```python
from build123d import *
from OCP.BRepAlgoAPI import BRepAlgoAPI_Cut
from OCP.TopTools import TopTools_ListOfShape

# Parameters (mm, degrees)
BOSS_EXTRUDE1_DEPTH = 75
FILLET1_R           = 2
SKETCH4_W           = 25.830037715
SKETCH4_H           = 76.964783177
CUT_EXTRUDE3_DEPTH  = 10
SKETCH7_W           = 75
SKETCH7_H           = 2.5
BOSS_EXTRUDE2_DEPTH = 7.180004
SKETCH9_W           = 2.5
SKETCH9_H           = 75
BOSS_EXTRUDE3_DEPTH = 20
SKETCH10_W          = 68.5
SKETCH10_H          = 2.5
BOSS_EXTRUDE4_DEPTH = 20
BOSS_EXTRUDE5_START = -67.82
BOSS_EXTRUDE5_DEPTH = 67.82
CUT_EXTRUDE4_DEPTH  = 7.32
SKETCH13_W          = 1.35
SKETCH13_H          = 15.1
CUT_EXTRUDE5_DEPTH  = 7.32
SKETCH15_R          = 1.15
CUT_EXTRUDE6_DEPTH  = 7.32
SKETCH16_R          = 1.15
CUT_EXTRUDE7_DEPTH  = 7.32
BOSS_EXTRUDE8_DEPTH = 59.999996
CHAMFER1_SIZE       = 0.75
CHAMFER2_SIZE       = 0.75


with BuildPart() as part:
    # Sketch1 → Boss-Extrude1 (new body)
    with BuildSketch(Plane(origin=(0, 0, 0), x_dir=(1, 0, 0), z_dir=(0, 1, 0))):
        with BuildLine():
            Line((-20.27294978, -55.394285714), (-17.826119678, -54.881428571))
            ThreePointArc((-17.826119678, -54.881428571), (-18.344064324, -51.565724334), (-18.517328344, -48.214285714))
            Line((-18.517328344, -48.214285714), (-18.517328344, 11.925714286))
            Line((-18.517328344, 11.925714286), (-5.357328344, 11.925714286))
            Line((-5.357328344, 11.925714286), (-5.357328344, 14.425714286))
            Line((-5.357328344, 14.425714286), (-21.017328344, 14.425714286))
            Line((-21.017328344, 14.425714286), (-21.017328344, -48.214285714))
            ThreePointArc((-21.017328344, -48.214285714), (-20.830736323, -51.823527305), (-20.27294978, -55.394285714))
        make_face()
    extrude(amount=BOSS_EXTRUDE1_DEPTH)

    # Fillet1
    fillet1_edges = [part.edges().sort_by_distance(p)[0] for p in [
        (-21.017328344, 37.5, -14.425714286),
        (-18.517328344, 37.5, -11.925714286),
    ]]
    fillet(fillet1_edges, radius=FILLET1_R)

    # Sketch4 → Cut-Extrude3 (cut)
    with BuildSketch(Plane(origin=(-18.517328344, 0, 0), x_dir=(0, 0, -1), z_dir=(1, 0, 0))):
        with Locations((-51.201481413, 38.482391589)):
            Rectangle(SKETCH4_W, SKETCH4_H)
    extrude(amount=CUT_EXTRUDE3_DEPTH, mode=Mode.SUBTRACT)

    # Sketch7 → Boss-Extrude2 (add)
    with BuildSketch(Plane(origin=(0, 0, 48.214285714), x_dir=(0, -1, 0), z_dir=(0, 0, 1))):
        with Locations((-37.5, -19.767328344)):
            Rectangle(SKETCH7_W, SKETCH7_H)
    extrude(amount=BOSS_EXTRUDE2_DEPTH)

    # Sketch9 → Boss-Extrude3 (add)
    with BuildSketch(Plane(origin=(-5.357328344, 0, 0), x_dir=(0, 0, -1), z_dir=(1, 0, 0))):
        with Locations((13.175714286, 37.5)):
            Rectangle(SKETCH9_W, SKETCH9_H)
    extrude(amount=BOSS_EXTRUDE3_DEPTH)

    # Sketch10 → Boss-Extrude4 (add)
    with BuildSketch(Plane(origin=(-18.517328344, 0, 0), x_dir=(0, 0, -1), z_dir=(1, 0, 0))):
        with Locations((-21.144285714, 73.75)):
            Rectangle(SKETCH10_W, SKETCH10_H)
    extrude(amount=BOSS_EXTRUDE4_DEPTH)

    # Sketch11 → Boss-Extrude5 (add)
    with BuildSketch(Plane.XY.offset(55.394285714).offset(BOSS_EXTRUDE5_START)):
        Polygon((-20.767328344, 0), (-18.767328344, 0), (-19.767328344, -2), align=None)
    extrude(amount=BOSS_EXTRUDE5_DEPTH)

    # Sketch12 → Cut-Extrude4 (cut)
    with BuildSketch(Plane.XY.offset(55.394285714)):
        Polygon((-20.767328344, 0), (-18.767328344, 0), (-19.767328344, -2), align=None)
    extrude(amount=-CUT_EXTRUDE4_DEPTH, mode=Mode.SUBTRACT)


with BuildPart() as cut_extrude5_tool:
    # Sketch13 → Cut-Extrude5 (new body)
    with BuildSketch(Plane.XY.offset(55.394285714)):
        with Locations((-20.342328344, 7.55)):
            Rectangle(SKETCH13_W, SKETCH13_H)
    extrude(amount=-CUT_EXTRUDE5_DEPTH)


with BuildPart() as part_1:
    add(part.part)

    # Cut-Extrude5: cut by cut_extrude5_tool, with a tolerance
    cut_extrude5_stock = TopTools_ListOfShape()
    cut_extrude5_stock.Append(part_1.part.wrapped)
    cut_extrude5_tools = TopTools_ListOfShape()
    cut_extrude5_tools.Append(cut_extrude5_tool.part.wrapped)
    cut_extrude5_cut = BRepAlgoAPI_Cut()
    cut_extrude5_cut.SetArguments(cut_extrude5_stock)
    cut_extrude5_cut.SetTools(cut_extrude5_tools)
    cut_extrude5_cut.SetFuzzyValue(0.00001)
    cut_extrude5_cut.Build()
    add(Compound.cast(cut_extrude5_cut.Shape()).solids(), mode=Mode.REPLACE)

    # Sketch15 → Cut-Extrude6 (cut)
    with BuildSketch(Plane(origin=(0, 0, -14.425714286), x_dir=(-1, 0, 0), z_dir=(0, 0, -1))):
        with Locations((-11.642671656, 64)):
            Circle(SKETCH15_R)
        with Locations((-11.642671656, 37.5)):
            Circle(SKETCH15_R)
        with Locations((-11.642671656, 11)):
            Circle(SKETCH15_R)
    extrude(amount=-CUT_EXTRUDE6_DEPTH, mode=Mode.SUBTRACT)

    # Sketch16 → Cut-Extrude7 (cut)
    with BuildSketch(Plane.ZY.offset(21.017328344)):
        with Locations((52.314285714, 64)):
            Circle(SKETCH16_R)
    extrude(amount=-CUT_EXTRUDE7_DEPTH, mode=Mode.SUBTRACT)

    # Sketch14 → Boss-Extrude8 (add)
    with BuildSketch(Plane.XY.offset(48.074285714)):
        Polygon((1.232671656, 75), (-0.767328344, 75), (0.232671656, 77), align=None)
    extrude(amount=-BOSS_EXTRUDE8_DEPTH)

    # Chamfer1
    chamfer1_edges = [part_1.edges().sort_by_distance(p)[0] for p in [
        (-21.017328344, 64, 51.164285714),
    ]]
    chamfer(chamfer1_edges, length=CHAMFER1_SIZE)

    # Chamfer2
    chamfer2_edges = [part_1.edges().sort_by_distance(p)[0] for p in [
        (12.792671656, 64, -14.425714286),
        (12.792671656, 37.5, -14.425714286),
        (12.792671656, 11, -14.425714286),
    ]]
    chamfer(chamfer2_edges, length=CHAMFER2_SIZE)


solid = part_1.part
```
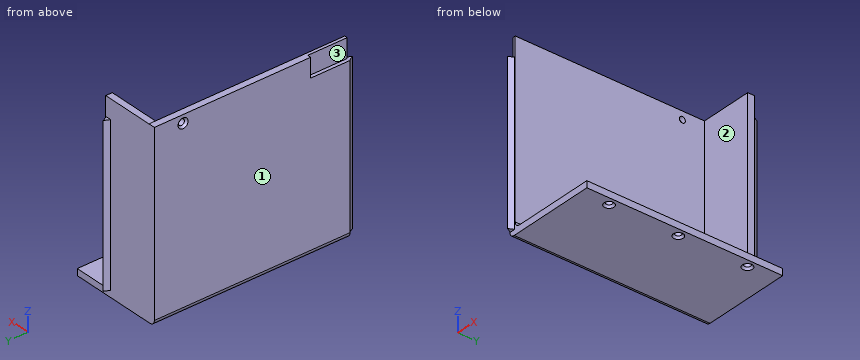
Work out the finished part from the listing and answer in its coordinate system (mm). Face numbers are marked on the shaded views. A direction names the side the tool comes from. Coordinates: 2 decimals unless noted, no trailing zeros. Loops run counter-clockwise (first coordinate to the right, second up) from the corner with the lowest first, then second, coordinate; pieces in that order, holes last. Notation, with made-up numbers: (40.25, 50) - (97.25, 50) arc R18 cw to (97.25, 67) - close; hole circle Ø4 at (59.5, -28). An arc over 180 degrees is marked (long way). Use a Markdown table: item, result.
Item 1: Find section A-A, the plane y = 11. Determine the outline of the cut face in (x, z), and give its area (3 significant figures).
Evaluation:
| item | result |
|---|---|
| outline | (-21.02, -12.43) arc R2 ccw to (-19.02, -14.43) - (9.74, -14.43) - (10.49, -13.68) - (10.49, -11.93) - (-16.52, -11.93) arc R2 cw to (-18.52, -9.93) - (-18.52, 55.39) - (-19.67, 55.39) - (-19.67, 48.07) - (-21.02, 48.07) - close; (12.79, -13.68) - (13.54, -14.43) - (14.64, -14.43) - (14.64, -11.93) - (12.79, -11.93) - close |
| area | 241 mm2 |
Item 2: Find section D-D, the plane x = -12. Determine the outline of the cut face in (y, z), and give its area (3 significant figures).
Evaluation:
| item | result |
|---|---|
| outline | (0, -14.43) - (75, -14.43) - (75, 55.39) - (72.5, 55.39) - (72.5, -11.93) - (0, -11.93) - close |
| area | 356 mm2 |
Item 3: Find section C-C, the plane z = 30.5. Determine the outline of the cut face in (x, y).
Evaluation:
| item | result |
|---|---|
| outline | (-21.02, 0) - (-20.77, 0) - (-19.77, -2) - (-18.77, 0) - (-18.52, 0) - (-18.52, 72.5) - (1.48, 72.5) - (1.48, 75) - (1.23, 75) - (0.23, 77) - (-0.77, 75) - (-21.02, 75) - close |
Item 4: Consider probe 1 along Z at (x, y) = (-19, 64); probe 2 along Y at (x, z) = (-4, 36.5); probe 3 along Z at (x, y) = (2, 42). Determine where each line is inside the solid, lowest interval first. Write a range as from..to.
Evaluation:
| item | result |
|---|---|
| probe 1 | z = -14.43..51.16, 53.46..55.39 |
| probe 2 | y = 72.5..75 |
| probe 3 | z = -14.43..-11.93 |
Item 5: Given pin 1 Ø0.8 at (y, z) = (73.5, 22) entering from +X; pin 2 Ø15.5 at (x, y) = (6, 34) entering from +Z; pin 3 Ø10.5 at (x, z) = (5, 22) entering from +Y; pin 4 Ø2 at (x, y) = (11.64, 37.5) entering from -Z, each flat-ended and moving along its own axis, determine where each tip first touches the part or whether it passes through.
Evaluation:
| item | result |
|---|---|
| pin 1 | stops at x = 1.48 |
| pin 2 | stops at z = -11.93 |
| pin 3 | stops at y = 77 |
| pin 4 | passes through |
Item 6: Find section B-B, the plane y = 64. Determine the outline of the cut face in (x, z).
Evaluation:
| item | result |
|---|---|
| outline | (-21.02, -12.43) arc R2 ccw to (-19.02, -14.43) - (9.74, -14.43) - (10.49, -13.68) - (10.49, -11.93) - (-16.52, -11.93) arc R2 cw to (-18.52, -9.93) - (-18.52, 51.16) - (-20.27, 51.16) - (-21.02, 50.41) - close; (-21.02, 54.21) - (-20.27, 53.46) - (-18.52, 53.46) - (-18.52, 55.39) - (-21.02, 55.39) - close; (12.79, -13.68) - (13.54, -14.43) - (14.64, -14.43) - (14.64, -11.93) - (12.79, -11.93) - close |
Item 7: For the marked faces 1, 2 and 3, determine the directions among +Z, -Z, +X, -X, +Y, -Y from which every point of the face is accessible in a straight line to the end or side of a thin tool.
Evaluation:
| item | result |
|---|---|
| face 1 | +Z, -Z, -X, +Y, -Y |
| face 2 | +Z, +X, -Y |
| face 3 | +Z, -X, -Y |
